Here's how the part is built. I have some questions about the finished solid (model axes, mm). A direction names the side the tool comes from. Give positions to 0.01 mm unless a question says otherwise; leave off trailing zeros. Order: outer loops, then holes, each group sorted by start corner. A loop starts at its lowest first (then second) coordinate and runs counter-clockwise, first axis right, second up.
Autodesk Inventor part; units mm, degrees
ref_plane "YZ Plane" through (0, 0, 0) normal (1, 0, 0) x (0, 1, 0)
ref_plane "XZ Plane" through (0, 0, 0) normal (0, 1, 0) x (-1, 0, 0)
ref_plane "XY Plane" through (0, 0, 0) normal (0, 0, 1) x (1, 0, 0)
sketch "Sketch1" plane through (0, 0, 0) normal (0, 0, 1) x (1, 0, 0)
  circle A0 centre (0, 17) radius 3.1
  line L0 (19.75, -8) -> (-19.75, -8)
  line L1 (19.75, 33) -> (19.75, -8)
  line L2 (-19.75, 33) -> (19.75, 33)
  line L3 (-19.75, -8) -> (-19.75, 33)
  line L4 (-19.75, -8) -> (19.75, -8)
  line L5 (19.75, -8) -> (19.75, -17)
  line L6 (19.75, -17) -> (-19.75, -17)
  line L7 (-19.75, -17) -> (-19.75, -8)
  line L8 (-19.75, 33) -> (19.75, 33)
  line L9 (19.75, 33) -> (19.75, 41)
  line L10 (19.75, 41) -> (-19.75, 41)
  line L11 (-19.75, 41) -> (-19.75, 33)
  line L12 (-19.75, -10) -> (19.75, -10)
  point P0 (0, 0)
  dimension "d0" = 7
  dimension "d1" = 8
extrude "Extrusion1" add sketch "Sketch1" along normal blind 17 contours A0 | L5 L12 L7 L0 | L0 L3 L2 L1 | L2 L11 L10 L9 | L5 L6 L7 L12
sketch "Sketch2" plane through (0, 0, 17) normal (0, 0, 1) x (1, 0, 0)
  line L0 (-19.75, -17) -> (19.75, -17)
  line L1 (-15, -17) -> (15, -17)
  line L2 (15, -17) -> (15, -12)
  line L3 (15, -12) -> (-15, -12)
  line L4 (-15, -12) -> (-15, -17)
  line L5 (0, 0) -> (0, 11.2749)
  point P0 (0, -12)
  dimension "d4" = 30
  dimension "d5" = 5
extrude "Extrusion2" add sketch "Sketch2" along normal blind 4.7
sketch "Sketch3" plane through (0, 0, 21.7) normal (0, 0, 1) x (1, 0, 0)
  line L0 (-15, -17) -> (15, -17)
  line L1 (15, -17) -> (15, -12)
  line L2 (15, -12) -> (-15, -12)
  line L3 (-15, -12) -> (-15, -17)
  line L4 (-28, -22) -> (28, -22)
  line L5 (28, -22) -> (28, 1)
  line L6 (28, 1) -> (-28, 1)
  line L7 (-28, 1) -> (-28, -22)
  line L8 (0, 0) -> (0, 8.1393)
  point P0 (0, 1)
  dimension "d8" = 56
  dimension "d9" = 23
  dimension "d10" = 5
extrude "Extrusion3" add sketch "Sketch3" along normal blind 32 contours L3 L2 L1 L0 | L7 L6 L5 L4
sketch "Sketch4" plane through (-28, -22, 21.7) normal (0, -1, 0) x (1, 0, 0)
  circle A0 centre (28, 16.697) radius 10.25
  point P0 (28, -21.7)
  dimension "d13" = 20.5
extrude "Extrusion4" add sketch "Sketch4" along normal blind 10.5
fillet "Fillet1" radius 3 12 edges at (-28, -10.5, 53.7) (28, -10.5, 53.7) (28, -10.5, 21.7) (-28, -10.5, 21.7) (-28, -22, 37.7) (0, -22, 21.7) (0, -22, 53.7) (28, -22, 37.7) (28, 1, 37.7) (-28, 1, 37.7) (0, 1, 53.7) (0, 1, 21.7)
sketch "Sketch5" plane through (0, -32.5, 38.397) normal (0, -1, 0) x (1, 0, 0)
  circle A0 centre (0, 0) radius 10.25
  circle A1 centre (0, 0) radius 7.1424
  point P0 (0, -38.397)
extrude "Extrusion5" cut sketch "Sketch5" against normal blind 1 contours A1
fillet "Fillet2" radius 1 2 edges at (15, -14.5, 17) (-15, -14.5, 17)
fillet "Fillet3" radius 4 2 edges at (0, 41, 0) (0, 41, 17)
properties part number "DK2 Camera"
Q1. If we section it at C-C on z = 27: List the corners of the cut face in (x, y) for me.
Filled sheet:
outline: (-28, -19) arc R3 ccw to (-25, -22) - (25, -22) arc R3 ccw to (28, -19) - (28, -2) arc R3 ccw to (25, 1) - (-25, 1) arc R3 ccw to (-28, -2) - close
Q2. For faces 1 (the face through (0, -17, 11)), 2 (the face through (15, -15, 20)), 3 (the face through (0, -12, 19)), 4 (the face through (19.75, 12, 8)), which set-ups out of +Z, -Z, +X, -X, +Y, -Y let a thin tool reach every point of the face, with its end or its side?
Filled sheet:
face 1: -Z, +X, -X, -Y
face 2: +X, +Y, -Y
face 3: +X, -X, +Y
face 4: -Z, +X, +Y, -Y
Q3. Thinking about a two-plate mould opening in Z: for faces 5 (the face through (0.35, -21.1, 52.84)), 6 (the face through (27.14, 0.1, 37.88)), 7 (the face through (-0.93, -32.01, 45.48)), which applies, released by +Z, released by -Z, zero draft, split by the parting line, or undercut?
Filled sheet:
face 5: released by +Z
face 6: zero draft
face 7: undercut
Q4. If we section it at A-A on y = -7.5: List the corners of the cut face in (x, z) for me.
Filled sheet:
outline: (-28, 24.7) arc R3 ccw to (-25, 21.7) - (25, 21.7) arc R3 ccw to (28, 24.7) - (28, 50.7) arc R3 ccw to (25, 53.7) - (-25, 53.7) arc R3 ccw to (-28, 50.7) - close; (-19.75, 0) - (19.75, 0) - (19.75, 17) - (-19.75, 17) - close
Q5. If we section it at D-D on y = 8: List the corners of the cut face in (x, z) for me.
Filled sheet:
outline: (-19.75, 0) - (19.75, 0) - (19.75, 17) - (-19.75, 17) - close
Q6. If we section it at B-B on x = 0: List the corners of the cut face in (y, z) for me, plus the area to 3 significant figures.
Filled sheet:
outline: (-32.5, 28.15) - (-22, 28.15) - (-22, 24.7) arc R3 ccw to (-19, 21.7) - (-17, 21.7) - (-17, 0) - (37, 0) arc R4 ccw to (41, 4) - (41, 13) arc R4 ccw to (37, 17) - (-12, 17) - (-12, 21.7) - (-2, 21.7) arc R3 ccw to (1, 24.7) - (1, 50.7) arc R3 ccw to (-2, 53.7) - (-19, 53.7) arc R3 ccw to (-22, 50.7) - (-22, 48.65) - (-32.5, 48.65) - (-32.5, 45.54) - (-31.5, 45.54) - (-31.5, 31.25) - (-32.5, 31.25) - close
area: 1,930 mm2
Q7. I'm going to push flat-ended pins straight in: P1, Ø10, axis at x = 20, z = 31, coming from the +Y side; P2, Ø5, axis at x = 14, z = 39, coming from the -Y side; P3, Ø1.5, axis at y = -2.5, z = 20.5, coming from the -X side; P4, Ø17.5, axis at x = -8.5, z = 7.5, coming from the -Y side. Where does each tip first touch, or does it pass through?
Filled sheet:
P1: stops at y = 1
P2: stops at y = -22
P3: passes through
P4: stops at y = -17
Q8. I need wall thicknesses on L1, parallel to Z at x = 18.5, y = -9; L2, parallel to X at y = -3.5, z = 7; L3, parallel to Y at x = 9, z = 49. Which ranges of each line are inside material? Lowest first, please.
Filled sheet:
L1: z = 0 to 17, 21.7 to 53.7
L2: x = -19.75 to 19.75
L3: y = -22 to 1
